Model file for the job. Use its own axes, mm. A direction names the side the tool comes from. Round coordinates to 2 decimals unless told otherwise and drop trailing zeros. Loops run counter-clockwise (first coordinate to the right, second up) from the corner with the lowest first, then second, coordinate; pieces in that order, holes last. Notation, with made-up numbers: (35.5, 70.25) - (55.5, 70.25) arc R16 cw to (55.5, 81.25) - close; hole circle Ø1 at (69, 60.5). An arc over 180 degrees is marked (long way). Use one line per item in the form item = value.
from build123d import *

# Parameters (mm, degrees)
SKETCH1_W                = 25
SKETCH1_H                = 25
SKETCH1_W_2              = 21
SKETCH1_H_2              = 21
BOSS_EXTRUDE1_DEPTH      = 375
SKETCH2_W                = 25
SKETCH2_H                = 25
BOSS_EXTRUDE2_DEPTH      = 2
SKETCH3_W                = 20
SKETCH3_H                = 20
SKETCH3_R                = 3.75
BOSS_EXTRUDE3_DEPTH      = 3
FILLET1_R                = 1
FILLET2_R                = 4
BOSS_EXTRUDE4_DEPTH      = 12.5
BOSS_EXTRUDE4_DEPTH_BACK = 12.5
CUT_EXTRUDE1_REACH       = 451.804
SKETCH5_W                = 21
SKETCH5_H                = 21
FILLET3_R                = 20
FILLET4_R                = 10
SKETCH6_W                = 25
SKETCH6_H                = 25
BOSS_EXTRUDE5_DEPTH      = 2
THICKEN1_START           = -12.5
THICKEN1_DEPTH           = 25
THICKEN2_START           = -12.5
THICKEN2_DEPTH           = 25
CUT_EXTRUDE2_DEPTH       = 482.455775371
CUT_EXTRUDE2_DEPTH_BACK  = 482.455775371
SKETCH9_R                = 3.75
FILLET6_R                = 4
FILLET7_R                = 5
CUT_EXTRUDE3_DEPTH       = 351.398422086
CUT_EXTRUDE3_DEPTH_BACK  = 351.398422086
SKETCH10_R               = 5


# Read off the part's stored shape, not the designer's step: Thicken1, Thicken2
with BuildPart() as part:
    # Sketch1 → Boss-Extrude1 (new body)
    with BuildSketch(Plane(origin=(0, 0, 0), x_dir=(0, 0, -1), z_dir=(1, 0, 0))):
        Rectangle(SKETCH1_W, SKETCH1_H)
        Rectangle(SKETCH1_W_2, SKETCH1_H_2, mode=Mode.SUBTRACT)
    extrude(amount=BOSS_EXTRUDE1_DEPTH)

    # Sketch2 → Boss-Extrude2 (add)
    with BuildSketch(Plane.ZY):
        Rectangle(SKETCH2_W, SKETCH2_H)
    extrude(amount=-BOSS_EXTRUDE2_DEPTH)

    # Sketch3 → Boss-Extrude3 (add, symmetric)
    with BuildSketch(Plane.XY):
        with Locations((-10, 0)):
            Rectangle(SKETCH3_W, SKETCH3_H)
        with Locations((-10, 0)):
            Circle(SKETCH3_R, mode=Mode.SUBTRACT)
    extrude(amount=BOSS_EXTRUDE3_DEPTH, both=True)

    # Fillet1
    fillet1_edges = [part.edges().sort_by_distance(p)[0] for p in [
        (0, 12.5, 0),
        (0, 0, -12.5),
        (0, 0, 3),
        (0, 0, -3),
        (0, -10, 0),
        (0, 10, 0),
        (0, -12.5, 0),
        (0, 0, 12.5),
    ]]
    fillet(fillet1_edges, radius=FILLET1_R)

    # Fillet2
    fillet2_edges = [part.edges().sort_by_distance(p)[0] for p in [
        (-20, 10, 0),
        (-20, -10, 0),
    ]]
    fillet(fillet2_edges, radius=FILLET2_R)

    # Sketch4 → Boss-Extrude4 (add, two sides: drawn at the far end of the back side and taken through both)
    with BuildSketch(Plane.XY.offset(-BOSS_EXTRUDE4_DEPTH_BACK)):
        Polygon((338.302222156, 12.5), (253.296790654, 246.050503583), (229.804475134, 237.5), (311.697777844, 12.5), align=None)
    extrude(amount=BOSS_EXTRUDE4_DEPTH + BOSS_EXTRUDE4_DEPTH_BACK)

    # Cut-Extrude1: up to this plane
    cut_extrude1_end = Plane(origin=(375, 10.5, -10.5), z_dir=(0, -1, 0))
    # Sketch5 → Cut-Extrude1 (cut, up to the surface)
    with BuildSketch(Plane(origin=(-49.449011673, 135.860042987, 0), x_dir=(0, 0, 1), z_dir=(-0.3420201433256653, 0.9396926207859098, 0)), mode=Mode.PRIVATE) as cut_extrude1_sk1:
        with Locations((0, 309.675353547)):
            Rectangle(SKETCH5_W, SKETCH5_H)
    cut_extrude1_tool1 = split(extrude(cut_extrude1_sk1.sketch, amount=-CUT_EXTRUDE1_REACH, mode=Mode.PRIVATE), bisect_by=cut_extrude1_end, keep=Keep.BOTH, mode=Mode.PRIVATE)
    add(cut_extrude1_tool1.solids().sort_by_distance((241.550633, 241.775252, 0))[0], mode=Mode.SUBTRACT)

    # Fillet3
    fillet3_edges = [part.edges().sort_by_distance(p)[0] for p in [
        (338.302222156, 12.5, 0),
    ]]
    fillet(fillet3_edges, radius=FILLET3_R)

    # Fillet4
    fillet4_edges = [part.edges().sort_by_distance(p)[0] for p in [
        (311.697777844, 12.5, 0),
    ]]
    fillet(fillet4_edges, radius=FILLET4_R)

    # Sketch6 → Boss-Extrude5 (add)
    with BuildSketch(Plane(origin=(375, 0, 0), x_dir=(0, 0, -1), z_dir=(1, 0, 0))):
        Rectangle(SKETCH6_W, SKETCH6_H)
    extrude(amount=-BOSS_EXTRUDE5_DEPTH)

    # Thicken1 outline → Thicken1 (add)
    with BuildSketch(Plane(origin=(0, 0, 0), x_dir=(1, 0, 0), z_dir=(0, 1, 0)).offset(THICKEN1_START)):
        Polygon((398.464101615, 3), (413.464101615, 3), (413.464101615, 5), (399, 5), (395.535898385, 7), (375, 7), (375, 5), (395, 5), align=None)
    extrude(amount=THICKEN1_DEPTH)

    # Thicken2 outline → Thicken2 (add)
    with BuildSketch(Plane(origin=(0, 0, 0), x_dir=(1, 0, 0), z_dir=(0, 1, 0)).offset(THICKEN2_START)):
        Polygon((399, -5), (413.464101615, -5), (413.464101615, -3), (398.464101615, -3), (395, -5), (375, -5), (375, -7), (395.535898385, -7), align=None)
    extrude(amount=THICKEN2_DEPTH)

    # Sketch9 → Cut-Extrude2 (cut, two sides: drawn at the far end of the back side and taken through both)
    with BuildSketch(Plane.XY.offset(5).offset(-CUT_EXTRUDE2_DEPTH_BACK)):
        with Locations(Location((406.232050808, 0, 0), (0, 0, 90))):
            Circle(SKETCH9_R)
    extrude(amount=CUT_EXTRUDE2_DEPTH + CUT_EXTRUDE2_DEPTH_BACK, mode=Mode.SUBTRACT)

    # Fillet6
    fillet6_edges = [part.edges().sort_by_distance(p)[0] for p in [
        (375, 0, -7),
        (395.535898385, 0, -7),
        (399, 0, -5),
        (375, 0, -5),
        (375, 0, 5),
        (375, 0, 7),
        (395.535898385, 0, 7),
        (399, 0, 5),
    ]]
    fillet(fillet6_edges, radius=FILLET6_R)

    # Fillet7
    fillet7_edges = [part.edges().sort_by_distance(p)[0] for p in [
        (413.464101615, 12.5, -4),
        (413.464101615, -12.5, -4),
        (413.464101615, 12.5, 4),
        (413.464101615, -12.5, 4),
    ]]
    fillet(fillet7_edges, radius=FILLET7_R)

    # Sketch10 → Cut-Extrude3 (cut, two sides: drawn at the far end of the back side and taken through both)
    with BuildSketch(Plane(origin=(302.745802327, 110.190460596, 0), x_dir=(0, 0, -1), z_dir=(0.9396926207859093, 0.34202014332566627, 0)).offset(-CUT_EXTRUDE3_DEPTH_BACK)):
        with Locations(Location((0, 124.579237914, 0), (0, 0, 90))):
            Circle(SKETCH10_R)
        with Locations(Location((0, 104.579237914, 0), (0, 0, 90))):
            Circle(SKETCH10_R)
        with Locations(Location((0, 84.579237914, 0), (0, 0, 90))):
            Circle(SKETCH10_R)
        with Locations(Location((0, 64.579237914, 0), (0, 0, 90))):
            Circle(SKETCH10_R)
        with Locations(Location((0, 44.579237914, 0), (0, 0, 90))):
            Circle(SKETCH10_R)
    extrude(amount=CUT_EXTRUDE3_DEPTH + CUT_EXTRUDE3_DEPTH_BACK, mode=Mode.SUBTRACT)


solid = part.part
1. Cut at B-B, the plane y = 126.5. Give the cut face in (x, z), plus the area to 3 significant figures.
Geometry check:
outline = (270.21, -12.5) - (296.81, -12.5) - (296.81, 12.5) - (270.21, 12.5) - close; hole (272.33, -10.5) - (294.68, -10.5) - (294.68, 10.5) - (272.33, 10.5) - close
area = 196 mm^2
2. Pull direction Z, two halves, no side cores. Call faces 1 (the flat face through (228, 3, 10.5)), 2 (the flat face through (387, 0, 7)), 3 (the flat face through (241.715, 241.835, 10.936)), 4 (the cylindrical face through (252.609, 177.727, -3.042)): +Z half, -Z half, draft (parallel to the pull), parting line (faces both ways), or undercut.
Geometry check:
face_1 = undercut
face_2 = +Z half
face_3 = draft
face_4 = undercut
3. Flat gauge pins, fed straight in: pin 1 (13 mm diameter, centred on x = 386.5, y = -4.5, fed in from -Z); pin 2 (1.6 mm diameter, centred on y = -1, z = 11.5, fed in from +X); pin 3 (12 mm diameter, centred on x = 218.5, z = 1.5, fed in from +Y). Where does each tip first touch, or does it go through?
Geometry check:
pin_1 = -7
pin_2 = 375.01
pin_3 = 12.5
4. Tool access for faces 5 (the flat face through (-15, 0, 3)), 6 (the flat face through (387, 0, -7)), 7 (the flat face through (403.7, -3, 5)), 8 (the flat face through (267.77, 133.19, -0.18)), 9 (the flat face through (272.539, 125.936, -0.147)): list every direction of +Z, -Z, +X, -X, +Y, -Y with a clear straight run to the whole face (end or side of a thin tool).
Geometry check:
face_5 = +Z, -X, +Y, -Y
face_6 = -Z, +X, +Y, -Y
face_7 = +Z, +X, +Y, -Y
face_8 = +Z, -Z, -X
face_9 = none
5. Cut at A-A, the plane x = 46. Give the cut face in (y, z), plus the area to 3 significant figures.
Geometry check:
outline = (-12.5, -12.5) - (12.5, -12.5) - (12.5, 12.5) - (-12.5, 12.5) - close; hole (-10.5, -10.5) - (10.5, -10.5) - (10.5, 10.5) - (-10.5, 10.5) - close
area = 184 mm^2
6. Wall check: probe 1 along Y at (x, z) = (50, 0.75); probe 2 along X at (y, z) = (0, -3.7); probe 3 along X at (y, z) = (0, 3.8). Give the ranges that are in metal, low to high.
Geometry check:
probe_1 = -12.5 to -10.5, 10.5 to 12.5
probe_2 = -0.05 to 2, 373 to 376.05, 397.25 to 402.48, 409.98 to 413.46
probe_3 = -0.02 to 2, 373 to 376.14, 397.08 to 402.48, 409.98 to 413.46
